from build123d import *

# Parameters (mm, degrees)
F0_R     = 1.75
F0_W     = 27.5
F0_H     = 42
F1_DEPTH = 4
F3_W     = 110
F3_H     = 73.4
F3_W_2   = 2
F3_H_2   = 55
F3_W_3   = 1
F4_DEPTH = 2
F5_SIZE  = 1
F6_DEPTH = 50
F9_DEPTH = 1
F10_R    = 5


# Not quite as in the source:
# - a feature names something its author has since deleted; it is built from what else it names


with BuildPart() as f1:
    # F0 (on Front) → F1 (new body)
    with BuildSketch(Plane.XZ):
        Polygon((-22.9204972982, 50.6646189876), (-72.9204972982, 50.6646189876), (-74.9204972982, 50.6646189876), (-74.9204972982, -24.3353810124), (-72.9204972982, -24.3353810124), (-22.9204972982, -24.3353810124), align=None)
        with Locations((-54.1704972982, -20.3353810124)):
            Circle(F0_R, mode=Mode.SUBTRACT)
        with Locations((-54.1704972982, 4.6646189876)):
            Rectangle(F0_W, F0_H, mode=Mode.SUBTRACT)
        with Locations((-54.1704972982, 29.6646189876)):
            Circle(F0_R, mode=Mode.SUBTRACT)
        with BuildLine():
            Line((-50.6704972982, 42.1646189876), (-50.6704972982, 47.1646189876))
            ThreePointArc((-50.6704972982, 47.1646189876), (-48.9204972982, 48.9146189876), (-47.1704972982, 47.1646189876))
            Line((-47.1704972982, 47.1646189876), (-47.1704972982, 42.1646189876))
            ThreePointArc((-47.1704972982, 42.1646189876), (-48.9204972982, 40.4146189876), (-50.6704972982, 42.1646189876))
        make_face(mode=Mode.SUBTRACT)
    extrude(amount=F1_DEPTH)

    # F3 (on line) → F4 (join, through all)
    with BuildSketch(Plane(origin=(-72.9204972982, 0, 0), x_dir=(0, -1, 0), z_dir=(-1, 0, 0))):
        with Locations((-55, 13.9646189876)):
            Rectangle(F3_W, F3_H)
        with Locations((-100, 13.1646189876)):
            Rectangle(F3_W_2, F3_H_2, mode=Mode.SUBTRACT)
        with Locations((-96, 13.1646189876)):
            Rectangle(F3_W_2, F3_H_2, mode=Mode.SUBTRACT)
        with Locations((-92, 13.1646189876)):
            Rectangle(F3_W_2, F3_H_2, mode=Mode.SUBTRACT)
        with Locations((-88, 13.1646189876)):
            Rectangle(F3_W_2, F3_H_2, mode=Mode.SUBTRACT)
        with Locations((-84, 13.1646189876)):
            Rectangle(F3_W_2, F3_H_2, mode=Mode.SUBTRACT)
        with Locations((-80, 13.1646189876)):
            Rectangle(F3_W_2, F3_H_2, mode=Mode.SUBTRACT)
        with Locations((-76, 13.1646189876)):
            Rectangle(F3_W_2, F3_H_2, mode=Mode.SUBTRACT)
        with Locations((-72, 13.1646189876)):
            Rectangle(F3_W_2, F3_H_2, mode=Mode.SUBTRACT)
        with Locations((-68, 13.1646189876)):
            Rectangle(F3_W_2, F3_H_2, mode=Mode.SUBTRACT)
        with Locations((-64, 13.1646189876)):
            Rectangle(F3_W_2, F3_H_2, mode=Mode.SUBTRACT)
        with Locations((-60, 13.1646189876)):
            Rectangle(F3_W_2, F3_H_2, mode=Mode.SUBTRACT)
        with Locations((-56, 13.1646189876)):
            Rectangle(F3_W_2, F3_H_2, mode=Mode.SUBTRACT)
        with Locations((-52, 13.1646189876)):
            Rectangle(F3_W_2, F3_H_2, mode=Mode.SUBTRACT)
        with Locations((-48, 13.1646189876)):
            Rectangle(F3_W_2, F3_H_2, mode=Mode.SUBTRACT)
        with Locations((-44, 13.1646189876)):
            Rectangle(F3_W_2, F3_H_2, mode=Mode.SUBTRACT)
        with Locations((-40, 13.1646189876)):
            Rectangle(F3_W_2, F3_H_2, mode=Mode.SUBTRACT)
        with Locations((-36, 13.1646189876)):
            Rectangle(F3_W_2, F3_H_2, mode=Mode.SUBTRACT)
        with Locations((-32, 13.1646189876)):
            Rectangle(F3_W_2, F3_H_2, mode=Mode.SUBTRACT)
        with Locations((-28, 13.1646189876)):
            Rectangle(F3_W_2, F3_H_2, mode=Mode.SUBTRACT)
        with Locations((-24, 13.1646189876)):
            Rectangle(F3_W_2, F3_H_2, mode=Mode.SUBTRACT)
        with Locations((-110.5, 13.9646189876)):
            Rectangle(F3_W_3, F3_H)
        Polygon((0, -24.3353810124), (0, -22.7353810124), (-110, -22.7353810124), (-111, -22.7353810124), (-111, -24.3353810124), align=None)
    extrude(amount=F4_DEPTH)

    # F5
    f5_edges = [f1.edges().sort_by_distance(p)[0] for p in [
        (-47.170497, -4, 44.664619),
    ]]
    chamfer(f5_edges, length=F5_SIZE)

    # F3 (on line) → F6 (join, through all)
    with BuildSketch(Plane(origin=(-72.9204972982, 0, 0), x_dir=(0, -1, 0), z_dir=(-1, 0, 0))):
        Polygon((0, -24.3353810124), (0, -22.7353810124), (-110, -22.7353810124), (-111, -22.7353810124), (-111, -24.3353810124), align=None)
    extrude(amount=-F6_DEPTH)

    # F8 (on line) → F9 (join, through all)
    with BuildSketch(Plane(origin=(0, 111, 0), x_dir=(-1, 0, 0), z_dir=(0, 1, 0))):
        with BuildLine():
            Line((64.9204972982, 16.4146189876), (72.9204972982, 16.4146189876))
            Line((72.9204972982, 16.4146189876), (72.9204972982, 28.9146189876))
            Line((72.9204972982, 28.9146189876), (64.9204972982, 28.9146189876))
            ThreePointArc((64.9204972982, 28.9146189876), (62.2688468688, 27.816269417), (61.1704972982, 25.1646189876))
            Line((61.1704972982, 25.1646189876), (61.1704972982, 20.1646189876))
            ThreePointArc((61.1704972982, 20.1646189876), (62.2688468688, 17.5129685581), (64.9204972982, 16.4146189876))
        make_face()
        with BuildLine():
            Line((63.1704972982, 20.1646189876), (63.1704972982, 25.1646189876))
            ThreePointArc((63.1704972982, 25.1646189876), (64.9204972982, 26.9146189876), (66.6704972982, 25.1646189876))
            Line((66.6704972982, 25.1646189876), (66.6704972982, 20.1646189876))
            ThreePointArc((66.6704972982, 20.1646189876), (64.9204972982, 18.4146189876), (63.1704972982, 20.1646189876))
        make_face(mode=Mode.SUBTRACT)
    extrude(amount=-F9_DEPTH)

    # F10
    f10_edges = [f1.edges().sort_by_distance(p)[0] for p in [
        (-22.920497, -2, 50.664619),
        (-73.920497, 111, 50.664619),
    ]]
    fillet(f10_edges, radius=F10_R)


solid = f1.part
Here's how the part is built. I have some questions about the finished solid (model axes, mm). A direction names the side the tool comes from. Coordinates: 2 decimals unless noted, no trailing zeros. Order: outer loops, then holes, each group sorted by start corner. A loop starts at its lowest first (then second) coordinate and runs counter-clockwise, first axis right, second up.
Item 1: For faces 5 (the face through (-62.24, 110.51, 17.54)), 6 (the face through (-62.298, 110.507, 27.845)), 7 (the face through (-47.17, -1, 45)), 8 (the face through (-67.92, -2, 4)), 9 (the face through (-74, 111, 0)), which set-ups out of +Z, -Z, +X, -X, +Y, -Y let a thin tool reach every point of the face, with its end or its side?
Result sheet:
face 5: +X, +Y, -Y
face 6: +Z, +X, +Y
face 7: +Y, -Y
face 8: -Y
face 9: +Z, -Z, +X, -X, +Y
Item 2: I need wall thicknesses on line 1 (Y direction, x = -28.5, z = 7.5); line 2 (Z direction, x = -53.5, y = 24); line 3 (X direction, y = 88.5, z = -18). Which ranges of each line are inside material? Lowest first, please.
Result sheet:
line 1: y = -4 to 0
line 2: z = -24.34 to -22.74
line 3: x = -74.92 to -72.92
Item 3: If we section it at A-A on x = -71: List the corners of the cut face in (y, z) for me.
Result sheet:
outline: (-4, -24.34) - (111, -24.34) - (111, -22.74) - (0, -22.74) - (0, 50.66) - (-4, 50.66) - close; (110, 16.41) - (111, 16.41) - (111, 28.91) - (110, 28.91) - close
Item 4: For P1, Ø4, axis at x = -54.17, z = 29.66, coming from the +Y side; P2, Ø1.5, axis at x = -62, y = 19, coming from the +Z side, each with a flat end and sliding along its axis, tell me the tip position at first contact or that it passes through.
Result sheet:
P1: stops at y = 0
P2: stops at z = -22.74
Item 5: If we mould it in two halves opening along Z, with no side actions, what happens to faces 1 (the face through (-67, 110, 23)), 2 (the face through (-48.879, -3.16, 40.255)), 3 (the face through (-48.959, -1.479, 48.914)), 4 (the face through (-73.934, 109.574, 49.161))? For each: +Z half, -Z half, draft (parallel to the pull), parting line (faces both ways), or undercut.
Result sheet:
face 1: draft
face 2: undercut
face 3: undercut
face 4: +Z half
Item 6: If we section it at B-B on z = 23.5: State how many separate pieces and enclosed holes the cut face has, plus the area to 3 significant figures.
Result sheet:
separate pieces: 23
enclosed holes: 0
area: 248 mm2
Item 7: If we section it at C-C on y = 15: List the corners of the cut face in (x, z) for me.
Result sheet:
outline: (-74.92, -24.34) - (-22.92, -24.34) - (-22.92, -22.74) - (-72.92, -22.74) - (-72.92, 50.66) - (-74.92, 50.66) - close
